Model file for the job. Use its own axes, mm. Face numbers are marked on the shaded views. A direction names the side the tool comes from. Coordinates: 2 decimals unless noted, no trailing zeros. Order: outer loops, then holes, each group sorted by start corner. A loop starts at its lowest first (then second) coordinate and runs counter-clockwise, first axis right, second up.
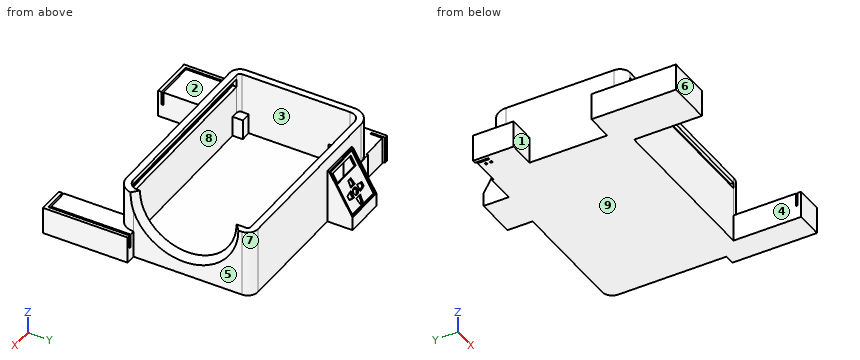
from build123d import *

# Parameters (mm, degrees)
SKETCH1_W           = 381
SKETCH1_H           = 254
BOSS_EXTRUDE1_DEPTH = 127
FILLET5_R           = 19.05
FILLET4_R           = 31.75
CUT_EXTRUDE1_DEPTH  = 114.3
CUT_EXTRUDE2_REACH  = 343.958
SKETCH5_W           = 330.2
SKETCH5_H           = 10.5
BOSS_EXTRUDE2_START = -50.8
BOSS_EXTRUDE2_DEPTH = 50.8
CUT_EXTRUDE3_DEPTH  = 25.4
BOSS_EXTRUDE3_DEPTH = 76.2
SKETCH10_W          = 71.12
SKETCH10_H          = 82.908181025
CUT_EXTRUDE4_DEPTH  = 12.7
CUT_EXTRUDE5_REACH  = 460.257
SKETCH11_W          = 71.12
SKETCH11_H          = 71.800590948
SKETCH12_W          = 71.12
SKETCH12_H          = 82.908181025
SKETCH12_R          = 6.35
SKETCH12_W_2        = 57.15
SKETCH12_H_2        = 19.05
BOSS_EXTRUDE4_DEPTH = 3.175
SKETCH13_W          = 330.2
SKETCH13_H          = 15.875
CUT_EXTRUDE6_DEPTH  = 7
SKETCH14_W          = 34.1
SKETCH14_H          = 66.2
CUT_EXTRUDE7_DEPTH  = 57.15
CUT_EXTRUDE8_START  = 34.1
CUT_EXTRUDE8_DEPTH  = 34.1
SKETCH16_W          = 11
SKETCH16_H          = 20
BOSS_EXTRUDE5_DEPTH = 5
SKETCH17_R          = 2
CUT_EXTRUDE9_DEPTH  = 367.998882862


# Read off the part's stored shape, not the designer's step: Boss-Extrude2
with BuildPart() as part:
    # Sketch1 → Boss-Extrude1 (new body)
    with BuildSketch(Plane.XY):
        Rectangle(SKETCH1_W, SKETCH1_H)
    extrude(amount=-BOSS_EXTRUDE1_DEPTH)

    # Fillet5
    fillet5_edges = [part.edges().sort_by_distance(p)[0] for p in [
        (-190.5, -127, -63.5),
        (190.5, 127, -63.5),
    ]]
    fillet(fillet5_edges, radius=FILLET5_R)

    # Fillet4
    fillet4_edges = [part.edges().sort_by_distance(p)[0] for p in [
        (190.5, -127, -63.5),
        (-190.5, 127, -63.5),
    ]]
    fillet(fillet4_edges, radius=FILLET4_R)

    # Sketch3 → Cut-Extrude1 (cut)
    with BuildSketch(Plane(origin=(0, 0, 0), x_dir=(-1, 0, 0), z_dir=(0, 0, -1))):
        with BuildLine():
            Line((-158.75, -114.3), (171.45, -114.3))
            ThreePointArc((171.45, -114.3), (175.940128061, -112.440128061), (177.8, -107.95))
            Line((177.8, -107.95), (177.8, 95.25))
            ThreePointArc((177.8, 95.25), (172.220384182, 108.720384182), (158.75, 114.3))
            Line((158.75, 114.3), (-171.45, 114.3))
            ThreePointArc((-171.45, 114.3), (-175.940128061, 112.440128061), (-177.8, 107.95))
            Line((-177.8, 107.95), (-177.8, -95.25))
            ThreePointArc((-177.8, -95.25), (-172.220384182, -108.720384182), (-158.75, -114.3))
        make_face()
    extrude(amount=CUT_EXTRUDE1_DEPTH, mode=Mode.SUBTRACT)

    # Sketch5 → Cut-Extrude2 (cut, up to next)
    with BuildSketch(Plane.XZ.offset(127), mode=Mode.PRIVATE) as cut_extrude2_sk1:
        with Locations((-6.35, -15.705)):
            Rectangle(SKETCH5_W, SKETCH5_H)
    cut_extrude2_tool1 = extrude(cut_extrude2_sk1.sketch, amount=-CUT_EXTRUDE2_REACH, mode=Mode.PRIVATE) & part.part
    add(cut_extrude2_tool1.solids().sort_by_distance((-6.35, -127, -15.705))[0], mode=Mode.SUBTRACT)

    # Sketch6 → Cut-Revolve1 (revolve, cut)
    with BuildSketch(Plane(origin=(0, 0, 0), x_dir=(1, 0, 0), z_dir=(0, 1, 0))):
        with BuildLine():
            Line((139.7, 0), (266.7, 0))
            Line((266.7, 0), (266.7, 127))
            ThreePointArc((266.7, 127), (176.897438789, 89.802561211), (139.7, 0))
        make_face()
    revolve(axis=Axis((266.7, 0, 0), (0, 0, -1)), mode=Mode.SUBTRACT)

    # Boss-Extrude2 outline → Boss-Extrude2 (add)
    with BuildSketch(Plane(origin=(0, 0, -127), x_dir=(-1, 0, 0), z_dir=(0, 0, -1)).offset(BOSS_EXTRUDE2_START)):
        with BuildLine():
            Line((-158.75, -254), (-158.75, -127))
            ThreePointArc((-158.75, -127), (-181.200640303, -117.700640303), (-190.5, -95.25))
            Line((-190.5, -95.25), (-209.55, -95.25))
            Line((-209.55, -95.25), (-209.55, -254))
            Line((-209.55, -254), (-158.75, -254))
        make_face()
        with BuildLine():
            ThreePointArc((-177.8, -95.25), (-172.220384182, -108.720384182), (-158.75, -114.3))
            Line((-158.75, -114.3), (-158.75, -95.25))
            Line((-158.75, -95.25), (-177.8, -95.25))
        make_face()
        with BuildLine():
            Line((158.75, -95.25), (158.75, -114.3))
            Line((158.75, -114.3), (171.45, -114.3))
            ThreePointArc((171.45, -114.3), (175.940128061, -112.440128061), (177.8, -107.95))
            Line((177.8, -107.95), (177.8, -95.25))
            Line((177.8, -95.25), (158.75, -95.25))
        make_face()
        with BuildLine():
            Line((241.3, -95.25), (190.5, -95.25))
            Line((190.5, -95.25), (190.5, -107.95))
            ThreePointArc((190.5, -107.95), (184.920384182, -121.420384182), (171.45, -127))
            Line((171.45, -127), (158.75, -127))
            Line((158.75, -127), (158.75, -254))
            Line((158.75, -254), (241.3, -254))
            Line((241.3, -254), (241.3, -95.25))
        make_face()
        with BuildLine():
            Line((241.3, 127), (234.95, 127))
            Line((234.95, 127), (234.95, 101.6))
            Line((234.95, 101.6), (231.775, 101.6))
            Line((231.775, 101.6), (231.775, 123.825))
            Line((231.775, 123.825), (180.975, 123.825))
            Line((180.975, 123.825), (180.975, 127))
            Line((180.975, 127), (158.75, 127))
            ThreePointArc((158.75, 127), (181.200640303, 117.700640303), (190.5, 95.25))
            Line((190.5, 95.25), (190.5, 50.8))
            Line((190.5, 50.8), (241.3, 50.8))
            Line((241.3, 50.8), (241.3, 127))
        make_face()
    extrude(amount=BOSS_EXTRUDE2_DEPTH)

    # Sketch8 → Cut-Extrude3 (cut)
    with BuildSketch(Plane.XY.offset(-76.2)):
        Polygon((-234.95, -95.25), (-234.95, -247.65), (-158.75, -247.65), (-158.75, -244.475), (-231.775, -244.475), (-231.775, -95.25), align=None)
        Polygon((158.75, -247.65), (203.2, -247.65), (203.2, -95.25), (200.025, -95.25), (200.025, -244.475), (158.75, -244.475), align=None)
    extrude(amount=-CUT_EXTRUDE3_DEPTH, mode=Mode.SUBTRACT)

    # Sketch9 → Boss-Extrude3 (add)
    with BuildSketch(Plane(origin=(-127, 0, 0), x_dir=(0, 0, -1), z_dir=(1, 0, 0))):
        Polygon((25.4, 127), (25.4, 130.175), (101.6, 174.169090512), (127, 174.169090512), (127, 127), align=None)
    extrude(amount=BOSS_EXTRUDE3_DEPTH)

    # Sketch10 → Cut-Extrude4 (cut)
    with BuildSketch(Plane(origin=(0, 86.632727372, 50.017428469), x_dir=(1, 0, 0), z_dir=(0, 0.866025403784436, 0.5000000000000047))):
        with Locations((-88.9, 131.078635769)):
            Rectangle(SKETCH10_W, SKETCH10_H)
    extrude(amount=-CUT_EXTRUDE4_DEPTH, mode=Mode.SUBTRACT)

    # Cut-Extrude5: up to this face of the body (flat: up to its plane)
    cut_extrude5_end = Plane(part.part.faces().sort_by_distance((-88.9, 141.173522628, -69.85))[0])
    # Sketch11 → Cut-Extrude5 (cut, up to the picked face)
    with BuildSketch(Plane.XZ.offset(-114.3), mode=Mode.PRIVATE) as cut_extrude5_sk1:
        with Locations((-88.9, -69.85)):
            Rectangle(SKETCH11_W, SKETCH11_H)
    cut_extrude5_tool1 = split(extrude(cut_extrude5_sk1.sketch, amount=-CUT_EXTRUDE5_REACH, mode=Mode.PRIVATE), bisect_by=cut_extrude5_end, keep=Keep.BOTH, mode=Mode.PRIVATE)
    add(cut_extrude5_tool1.solids().sort_by(Axis((-88.9, 114.3, -69.85), (0, 1, 0)))[0], mode=Mode.SUBTRACT)

    # Sketch12 → Boss-Extrude4 (add)
    with BuildSketch(Plane(origin=(0, 83.883096715, 48.429928469), x_dir=(1, 0, 0), z_dir=(0, 0.866025403784436, 0.5000000000000047))):
        with Locations((-88.9, 131.078635769)):
            Rectangle(SKETCH12_W, SKETCH12_H)
        with Locations(Location((-88.9, 147.132726281, 0), (0, 0, 270))):
            Circle(SKETCH12_R, mode=Mode.SUBTRACT)
        Polygon((-82.55, 136.972726281), (-95.25, 136.972726281), (-92.71, 124.272726281), (-85.09, 124.272726281), align=None, mode=Mode.SUBTRACT)
        Polygon((-78.74, 153.482726281), (-66.04, 150.942726281), (-66.04, 143.322726281), (-78.74, 140.782726281), align=None, mode=Mode.SUBTRACT)
        Polygon((-99.06, 140.782726281), (-99.06, 153.482726281), (-111.76, 150.942726281), (-111.76, 143.322726281), align=None, mode=Mode.SUBTRACT)
        Polygon((-95.25, 157.292726281), (-82.55, 157.292726281), (-85.09, 169.992726281), (-92.71, 169.992726281), align=None, mode=Mode.SUBTRACT)
        with Locations((-88.265, 105.499545256)):
            Rectangle(SKETCH12_W_2, SKETCH12_H_2, mode=Mode.SUBTRACT)
    extrude(amount=-BOSS_EXTRUDE4_DEPTH)

    # Sketch13 → Cut-Extrude6 (cut)
    with BuildSketch(Plane(origin=(0, -114.3, 0), x_dir=(1, 0, 0), z_dir=(0, 1, 0))):
        with Locations((-6.35, 15.955)):
            Rectangle(SKETCH13_W, SKETCH13_H)
    extrude(amount=-CUT_EXTRUDE6_DEPTH, mode=Mode.SUBTRACT)

    # Sketch14 → Cut-Extrude7 (cut)
    with BuildSketch(Plane(origin=(-234.95, 0, 0), x_dir=(0, 0, -1), z_dir=(1, 0, 0))):
        with Locations((97.25, 87.9)):
            Rectangle(SKETCH14_W, SKETCH14_H)
    extrude(amount=CUT_EXTRUDE7_DEPTH, mode=Mode.SUBTRACT)

    # Sketch15 → Cut-Extrude8 (cut)
    with BuildSketch(Plane.XY.offset(-114.3).offset(CUT_EXTRUDE8_START)):
        with BuildLine():
            Line((-158.75, 114.3), (-177.8, 114.3))
            Line((-177.8, 114.3), (-177.8, 95.25))
            ThreePointArc((-177.8, 95.25), (-172.220384182, 108.720384182), (-158.75, 114.3))
        make_face()
    extrude(amount=-CUT_EXTRUDE8_DEPTH, mode=Mode.SUBTRACT)

    # Sketch16 → Boss-Extrude5 (add)
    with BuildSketch(Plane.XY.offset(-114.3)):
        with Locations((-226.275, 108)):
            Rectangle(SKETCH16_W, SKETCH16_H)
    extrude(amount=BOSS_EXTRUDE5_DEPTH)

    # Sketch17 → Cut-Extrude9 (cut, through all)
    with BuildSketch(Plane.XY.offset(-109.3)):
        with Locations((-223.675, 112.5)):
            Circle(SKETCH17_R)
        with Locations((-223.675, 103)):
            Circle(SKETCH17_R)
    extrude(amount=-CUT_EXTRUDE9_DEPTH, mode=Mode.SUBTRACT)


solid = part.part
Q1. Which spindle directions (+Z, -Z, +X, -X, +Y, -Y) get a long thin tool onto all of the face, cutting with end or side? Do the marked faces 1, 2, 3, 4 and 5. Say none if no direction does.
Established:
face 1: +Z, -Z, -X
face 2: +Z, -X, -Y
face 3: +Z
face 4: +Z, -Z, -Y
face 5: +Z, -Z, +X, +Y
Q2. Probe line 1 (X direction, y = -219.5, z = -88.5) (3 decimals); line 2 (Y direction, x = 40.5, z = -93.5); line 3 (X direction, y = 138.5, z = -48.5). List the from-to ranges inside material, lowest first.
Established:
line 1: x = -241.3 to -234.95, -231.775 to -158.75, 158.75 to 200.025, 203.2 to 209.55
line 2: y = -127 to -114.3, 114.3 to 127
line 3: x = -127 to -116.84, -59.69 to -50.8
Q3. Drop flat-ended pins along their axis: P1, Ø2.5, axis at y = 154.5, z = -82, coming from the +X side; P2, Ø5.5, axis at y = 106, z = -111, coming from the +X side; P3, Ø1, axis at x = 53.5, z = -108.5, coming from the +Y side. Give the stop position or say it passes through.
Established:
P1: stops at x = -50.8
P2: stops at x = 190.5
P3: stops at y = 127
Q4. Cut at C-C, the plane y = -15. List the corners of the cut face in (x, z), plus the area to 3 significant figures.
Established:
outline: (-190.5, -127) - (190.5, -127) - (190.5, -100.49) arc R126.11 cw to (177.8, -89.45) - (177.8, -114.3) - (-177.8, -114.3) - (-177.8, 0) - (-190.5, 0) - close
area: 6,530 mm2
Q5. Cut at A-A, the plane x = -15. List the corners of the cut face in (y, z) (1 decimal).
Established:
outline: (-127, -127) - (127, -127) - (127, 0) - (114.3, 0) - (114.3, -114.3) - (-114.3, -114.3) - (-114.3, -23.9) - (-121.3, -23.9) - (-121.3, -21) - (-127, -21) - close; (-127, -10.5) - (-121.3, -10.5) - (-121.3, -8) - (-114.3, -8) - (-114.3, 0) - (-127, 0) - close
Q6. Cut at B-B, the plane y = 41.5. List the corners of the cut face in (x, z), plus the area to 3 significant figures.
Established:
outline: (-190.5, -127) - (190.5, -127) - (190.5, -92.74) arc R120.03 cw to (177.8, -80.64) - (177.8, -114.3) - (-177.8, -114.3) - (-177.8, 0) - (-190.5, 0) - close
area: 6,640 mm2
Q7. Mould opens along Y. For the marked faces 6, 7, 8 and 9 say: pulls with the +Y half, pulls with the -Y half, needs draft (parallel to the pull), parting line crosses it, or undercut.
Established:
face 6: pulls with the -Y half
face 7: pulls with the +Y half
face 8: undercut
face 9: needs draft
